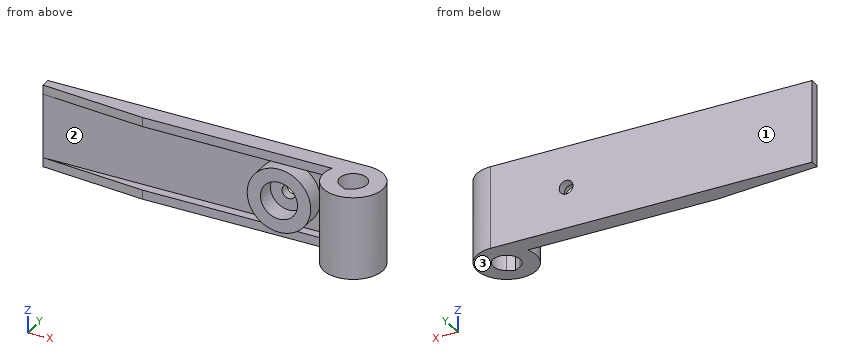
```python
from build123d import *

# Parameters (mm, degrees)
MAIN_DEPTH          = 9
RIB_START           = -7
RIB_DEPTH           = 2
BOSS_EXTRUDE1_START = 9
BOSS_EXTRUDE1_DEPTH = 2
SKETCH2_R           = 1.5
CUT_EXTRUDE1_DEPTH  = 72.656236938
BOSS_EXTRUDE2_START = 4
SKETCH2_4_R         = 6.95
SKETCH2_4_R_2       = 4.05
SKETCH2_4_R_3       = 1.5
BOSS_EXTRUDE2_DEPTH = 4


with BuildPart() as part:
    # Sketch1 → main (new, symmetric)
    with BuildSketch(Plane.XY):
        with BuildLine():
            Line((0, 6.475), (-70.2404, 6.475))
            Line((-70.2404, 6.475), (-70.2404, 4.475))
            Line((-70.2404, 4.475), (-4.679743583, 4.475))
            ThreePointArc((-4.679743583, 4.475), (2.54460213, -5.954042744), (0, 6.475))
        make_face()
        with BuildLine():
            Line((1.4875, -2.576425576), (0, -3.435234102))
            Line((0, -3.435234102), (-1.4875, -2.576425576))
            ThreePointArc((-1.4875, -2.576425576), (0, 2.975), (1.4875, -2.576425576))
        make_face(mode=Mode.SUBTRACT)
    extrude(amount=MAIN_DEPTH, both=True)

    # Sketch1<4> → rib (add)
    with BuildSketch(Plane.XY.offset(RIB_START)):
        with BuildLine():
            Line((-47.380295394, 2.475), (-5.983310121, 2.475))
            ThreePointArc((-5.983310121, 2.475), (-5.424498002, 3.53559704), (-4.679743583, 4.475))
            Line((-4.679743583, 4.475), (-70.2404, 4.475))
            Line((-70.2404, 4.475), (-47.380295394, 2.475))
        make_face()
    extrude(amount=-RIB_DEPTH)

    # Sketch1<5> → Boss-Extrude1 (add)
    with BuildSketch(Plane.XY.offset(BOSS_EXTRUDE1_START)):
        with BuildLine():
            Line((-47.380295394, 2.475), (-5.983310121, 2.475))
            ThreePointArc((-5.983310121, 2.475), (-5.424498002, 3.53559704), (-4.679743583, 4.475))
            Line((-4.679743583, 4.475), (-70.2404, 4.475))
            Line((-70.2404, 4.475), (-47.380295394, 2.475))
        make_face()
    extrude(amount=-BOSS_EXTRUDE1_DEPTH)

    # Sketch2 → Cut-Extrude1 (cut, through all)
    with BuildSketch(Plane.XZ.offset(-4.475)):
        with Locations((-16.5, 0)):
            Circle(SKETCH2_R)
    extrude(amount=-CUT_EXTRUDE1_DEPTH, mode=Mode.SUBTRACT)

    # Sketch2<4> → Boss-Extrude2 (add)
    # profile 1 of 2: a face of its own
    with BuildSketch(Plane.XZ.offset(-4.475).offset(BOSS_EXTRUDE2_START)):
        with Locations(Location((-16.5, 0, 0), (0, 0, 180))):
            Circle(SKETCH2_4_R)
        with Locations((-16.5, 0)):
            Circle(SKETCH2_4_R_2, mode=Mode.SUBTRACT)
    # profile 2 of 2: a face of its own
    with BuildSketch(Plane.XZ.offset(-4.475).offset(BOSS_EXTRUDE2_START)):
        with Locations((-16.5, 0)):
            Circle(SKETCH2_4_R_3)
    extrude(amount=-BOSS_EXTRUDE2_DEPTH)


with BuildPart() as boss_extrude2_kept_piece:
    # of the separate pieces the step leaves, the one the design keeps (boss_extrude2_pieces_kept)
    add(part.part.solids().sort_by_distance((0, 6.475, -9))[0])


solid = boss_extrude2_kept_piece.part
```
Work out the finished part from the listing and answer in its coordinate system (mm). Face numbers are marked on the shaded views. Coordinates: 2 decimals unless noted, no trailing zeros. Order: outer loops, then holes, each group sorted by start corner. A loop starts at its lowest first (then second) coordinate and runs counter-clockwise, first axis right, second up. Notation, with made-up numbers: (69, 74) - (93, 74) arc R28 cw to (93, 95) - close; hole circle Ø2 at (87, -12.75). An arc over 180 degrees is marked (long way). Answer as a JSON object with one key per item and string values.
1. Find section B-B on x = -16.5. Determine the outline of the cut face in (y, z) (3 decimals).
Output values:
{"outline": "(0.475, -6.95) - (4.475, -6.95) - (4.475, -7) - (2.475, -7) - (2.475, -9) - (6.475, -9) - (6.475, -1.5) - (4.475, -1.5) - (4.475, -4.05) - (0.475, -4.05) - close; (0.475, 4.05) - (4.475, 4.05) - (4.475, 1.5) - (6.475, 1.5) - (6.475, 9) - (2.475, 9) - (2.475, 7) - (4.475, 7) - (4.475, 6.95) - (0.475, 6.95) - close"}
2. Consider line 1 (Z direction, x = -52, y = 3); line 2 (Y direction, x = -54, z = 6) (3 decimals); line 3 (X direction, y = -0.25, z = 6.25). Determine where each line is inside the solid, lowest interval first.
Output values:
{"line 1": "z = -9 to -7, 7 to 9", "line 2": "y = 4.475 to 6.475", "line 3": "x = -6.47 to -2.96, 2.96 to 6.47"}
3. Each of these flat-tipped pins is pushed along its axis until it touches: P1, Ø7, axis at x = -14.5, z = 0.5, coming from the -Y side (3 decimals); P2, Ø2.5, axis at x = -16.5, z = 1, coming from the -Y side (3 decimals); P3, Ø1.6, axis at x = -17.5, z = 8, coming from the -Y side (3 decimals). Where does it stop, or does it pass through?
Output values:
{"P1": "stops at y = 0.475", "P2": "stops at y = 4.475", "P3": "stops at y = 2.475"}
4. The mould has two halves that part along Z. Classify the marked faces 1, 2 and 3: +Z half, -Z half, draft (parallel to the pull), parting line (faces both ways), or undercut.
Output values:
{"face 1": "draft", "face 2": "undercut", "face 3": "-Z half"}
5. Find section C-C on y = 3.75. Determine the outline of the cut face in (x, z), plus the area to 3 significant figures.
Output values:
{"outline": "(-61.95, -9) - (5.28, -9) - (5.28, 9) - (-61.95, 9) - (-61.95, 7) - (-5.28, 7) - (-5.28, -7) - (-61.95, -7) - close; circle Ø13.9 at (-16.5, 0); hole circle Ø8.1 at (-16.5, 0)", "area": "517 mm²"}
6. Find section A-A on z = 0. Count the separate pieces of the cut face and the enclosed holes in it, plus the area to 3 significant figures.
Output values:
{"separate pieces": "2", "enclosed holes": "1", "area": "255 mm²"}
7. Find section D-D on x = -24.5. Determine the outline of the cut face in (y, z) (3 decimals).
Output values:
{"outline": "(2.475, -9) - (6.475, -9) - (6.475, 9) - (2.475, 9) - (2.475, 7) - (4.475, 7) - (4.475, -7) - (2.475, -7) - close"}
